The listing builds one solid part. Answer for the finished solid, in the listing's coordinates (mm). A direction names the side the tool comes from. Give positions to 0.01 mm unless a question says otherwise; leave off trailing zeros. Loops run counter-clockwise (first coordinate to the right, second up) from the corner with the lowest first, then second, coordinate; pieces in that order, holes last.
Item 1: Section B-B, the plane x = -79 is taken. Give the vertices of the cut face in (y, z), and give its area (3 significant figures).
Item 2: Consider line 1 along Z through (x, y) = (253.75, 1.55); line 2 along X through (y, z) = (1.95, 368.75); line 3 along X through (y, z) = (2.4, 371). Determine where each line is inside the solid, lowest interval first.
Item 3: This flat-tipped pin is pushed along its axis until it touches: pin 1 Ø2 at (x, z) = (-183.75, 343.75) entering from -Y. Where does it stop, or does it pass through?
Item 4: The mould has two halves that part along Z. Classify faces 3 (the face through (233.986, 2.028, 349.297)), 4 (the face through (253, 4, 76)): pulls with the +Z half, pulls with the -Z half, needs draft (parallel to the pull), parting line crosses it, or undercut.
Item 5: Section C-C, the plane y = 1.95 is taken. Give the number of separate pieces and of enclosed holes in the cut face, and give its area (3 significant figures).
Item 6: A tool of negligible diameter and unlimited length cuts with its end or side. For faces 1 (the face through (234.297, 2.028, -198.986)), 2 (the face through (253, 0, 76)), from which of +Z, -Z, +X, -X, +Y, -Y can it reach the whole face along a straight path? Write none if from no direction.
Item 7: Section A-A, the plane z = 162 is taken. Give the vertices of the cut face in (x, y).
Autodesk Inventor part; units mm, degrees
ref_plane "YZ Plane" through (0, 0, 0) normal (1, 0, 0) x (0, 1, 0)
ref_plane "XZ Plane" through (0, 0, 0) normal (0, 1, 0) x (-1, 0, 0)
ref_plane "XY Plane" through (0, 0, 0) normal (0, 0, 1) x (1, 0, 0)
sketch "Эскиз1" plane through (0, 0, 0) normal (0, 1, 0) x (-1, 0, 0)
  line L0 (-260, 375) -> (190, 375)
  line L1 (190, 375) -> (190, -225)
  line L2 (190, -225) -> (-260, -225)
  line L3 (-260, -225) -> (-260, 375)
  line L4 (-260, 375) -> (190, -225) construction
  line L5 (190, 375) -> (-260, -225) construction
  circle A0 centre (-228.75, 368.75) radius 1.75
  circle A1 centre (-253.75, 343.75) radius 1.75
  circle A2 centre (-256, 371) radius 1.75
  circle A3 centre (186, 371) radius 1.75
  circle A4 centre (183.75, 343.75) radius 1.75
  circle A5 centre (158.75, 368.75) radius 1.75
  circle A6 centre (183.75, -193.75) radius 1.75
  circle A7 centre (186, -221) radius 1.75
  circle A8 centre (158.75, -218.75) radius 1.75
  circle A9 centre (-253.75, -193.75) radius 1.75
  circle A10 centre (-256, -221) radius 1.75
  circle A11 centre (-228.75, -218.75) radius 1.75
  line L6 (170, -205) -> (170, 355)
  line L7 (170, 355) -> (-240, 355)
  line L8 (-240, 355) -> (-240, -205)
  line L9 (-240, -205) -> (170, -205)
  point P0 (0, 0)
  dimension "d0" = 450
  dimension "d1" = 600
  dimension "d11" = 20
  dimension "d21" = 27.25
  dimension "d22" = 2.25
  dimension "d23" = 27.25
  dimension "d24" = 2.25
  dimension "d25" = 4
  dimension "d26" = 4
  dimension "d27" = 27.25
  dimension "d28" = 4
  dimension "d29" = 4
  dimension "d30" = 27.25
  dimension "d31" = 2.25
  dimension "d32" = 2.25
  dimension "d34" = 27.25
  dimension "d35" = 27.25
  dimension "d36" = 2.25
  dimension "d37" = 2.25
  dimension "d38" = 4
  dimension "d39" = 4
  dimension "d40" = 27.25
  dimension "d41" = 27.25
  dimension "d42" = 2.25
  dimension "d43" = 2.25
  dimension "d44" = 4
  dimension "d45" = 4
extrude "Выдавливание1" add sketch "Эскиз1" along normal blind 4
fillet "Сопряжение1" radius 20 4 edges at (240, 2, -205) (-170, 2, -205) (-170, 2, 355) (240, 2, 355)
sketch "Эскиз2" plane through (0, 4, 0) normal (0, 1, 0) x (1, 0, 0)
  circle A0 centre (-177.5, 212.5) radius 7
  circle A1 centre (247.5, 212.5) radius 7
  circle A2 centre (247.5, -362.5) radius 7
  circle A3 centre (-177.5, -362.5) radius 7
  circle A4 centre (-177.5, -362.5) radius 5
  circle A5 centre (247.5, -362.5) radius 5
  circle A6 centre (247.5, 212.5) radius 5
  circle A7 centre (-177.5, 212.5) radius 5
  line L0 (260, 225) -> (-190, 225)
  point P0 (0, 0)
  dimension "d15" = 10
  dimension "d16" = 10
  dimension "d17" = 10
  dimension "d18" = 10
  dimension "d33" = 12.5
extrude "Выдавливание2" cut sketch "Эскиз2" against normal through all contours A4 | A5 | A6 | A7
properties part number "top_plate"
Worked answers:
1. outline: (0, -225) - (4, -225) - (4, -205) - (0, -205) - close; (0, 355) - (4, 355) - (4, 375) - (0, 375) - close
1. area: 160 mm2
2. line 1: z = -225 to -195.5, -192 to 342, 345.5 to 375
2. line 2: x = -190 to -160.5, -157 to 227, 230.5 to 260
2. line 3: x = -190 to -187.75, -184.25 to 254.25, 257.75 to 260
3. pin 1: passes through
4. face 3: undercut
4. face 4: needs draft
5. separate pieces: 1
5. enclosed holes: 17
5. area: 40,300 mm2
6. face 1: +Y, -Y
6. face 2: +Z, -Z, +X, -X, -Y
7. outline: (-190, 0) - (-170, 0) - (-170, 4) - (-190, 4) - close; (240, 0) - (260, 0) - (260, 4) - (240, 4) - close
